Source: CAD feature listing. Evaluate the final solid. Frame: model axes, mm. Face numbers are marked on the shaded views. Round coordinates to 2 decimals unless told otherwise and drop trailing zeros. Loops run counter-clockwise (first coordinate to the right, second up) from the corner with the lowest first, then second, coordinate; pieces in that order, holes last.
Item 1: First-contact query: P1, Ø3, axis at y = -28.5, z = -3, coming from the +X side; P2, Ø8, axis at x = -10.5, y = -26, coming from the +Z side; P3, Ø3, axis at x = 9, y = -29, coming from the +Z side. Flat tips, straight axial feed; report the tip coordinate or a pass-through.
Item 2: Section query A-A on z = 0. Return loops of the section in (x, y).
Item 3: Section query B-B on x = 0. Return loops of the section in (y, z).
Item 4: Section query C-C on y = -27.5. Return loops of the section in (x, z).
Item 5: Pull-direction query (Z, two-part tool) for the marked faces 1, 2 and 3; classes: released by +Z, released by -Z, zero draft, split by the parting line, or undercut.
Item 6: Ray query, L1, parallel to X at y = -27.75, z = 0; L2, parallel to X at y = -24.5, z = 16. Return the intervals inside material, ascending.
```python
from build123d import *

# Parameters (mm, degrees)
RACCORDO1_R  = 4
SMUSSO1_SIZE = 0.5
SMUSSO2_SIZE = 0.3
RACCORDO5_R  = 0.8


with BuildPart() as part:
    # Schizzo1 → Rivoluzione1 (revolve)
    with BuildSketch(Plane.XY):
        Polygon((-34, -19.165655205), (-34, -34.165655205), (-23.25, -34.165655205), (-22.25, -33.465655205), (-20, -33.465655205), (-20, -20.665655205), (-17.75, -20.665655205), (-17.75, -19.165655205), align=None)
    revolve(axis=Axis((0, 44.110898502, 0), (0, -1, 0)))

    # Raccordo1
    raccordo1_edges = [part.edges().sort_by_distance(p)[0] for p in [
        (34, -34.165655205, 0),
        (34, -19.165655205, 0),
    ]]
    fillet(raccordo1_edges, radius=RACCORDO1_R)

    # Smusso1
    smusso1_edges = [part.edges().sort_by_distance(p)[0] for p in [
        (17.75, -19.165655205, 0),
    ]]
    chamfer(smusso1_edges, length=SMUSSO1_SIZE)

    # Smusso2
    smusso2_edges = [part.edges().sort_by_distance(p)[0] for p in [
        (20, -33.465655205, 0),
    ]]
    chamfer(smusso2_edges, length=SMUSSO2_SIZE)

    # Raccordo5
    raccordo5_edges = [part.edges().sort_by_distance(p)[0] for p in [
        (20, -20.665655205, 0),
    ]]
    fillet(raccordo5_edges, radius=RACCORDO5_R)


solid = part.part
```
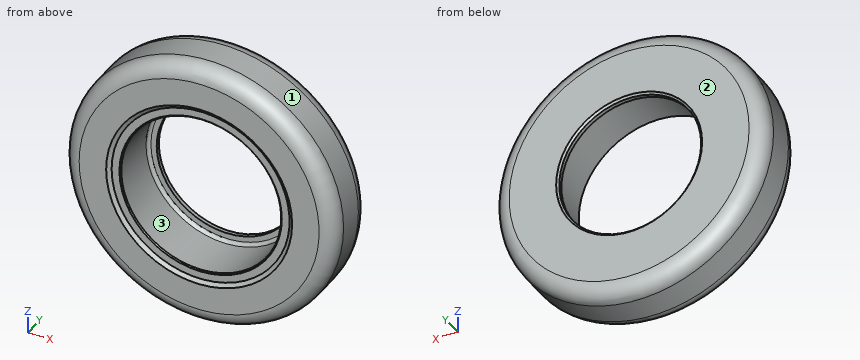
Data:
1. P1: stops at x = 33.97
1. P2: stops at z = 33.37
1. P3: stops at z = 33.16
2. outline: (-34, -30.17) arc R4 ccw to (-30, -34.17) - (-23.25, -34.17) - (-22.25, -33.47) - (-20.3, -33.47) - (-20, -33.17) - (-20, -21.47) arc R0.8 cw to (-19.2, -20.67) - (-17.75, -20.67) - (-17.75, -19.67) - (-18.25, -19.17) - (-30, -19.17) arc R4 ccw to (-34, -23.17) - close; (17.75, -20.67) - (19.2, -20.67) arc R0.8 cw to (20, -21.47) - (20, -33.17) - (20.3, -33.47) - (22.25, -33.47) - (23.25, -34.17) - (30, -34.17) arc R4 ccw to (34, -30.17) - (34, -23.17) arc R4 ccw to (30, -19.17) - (18.25, -19.17) - (17.75, -19.67) - close
3. outline: (-34.17, -30) arc R4 ccw to (-30.17, -34) - (-23.17, -34) arc R4 ccw to (-19.17, -30) - (-19.17, -18.25) - (-19.67, -17.75) - (-20.67, -17.75) - (-20.67, -19.2) arc R0.8 cw to (-21.47, -20) - (-33.17, -20) - (-33.47, -20.3) - (-33.47, -22.25) - (-34.17, -23.25) - close; (-34.17, 23.25) - (-33.47, 22.25) - (-33.47, 20.3) - (-33.17, 20) - (-21.47, 20) arc R0.8 cw to (-20.67, 19.2) - (-20.67, 17.75) - (-19.67, 17.75) - (-19.17, 18.25) - (-19.17, 30) arc R4 ccw to (-23.17, 34) - (-30.17, 34) arc R4 ccw to (-34.17, 30) - close
4. outline: circle Ø68 at (0, 0); hole circle Ø40 at (0, 0)
5. face 1: split by the parting line
5. face 2: zero draft
5. face 3: undercut
6. L1: x = -34 to -20, 20 to 34
6. L2: x = -30 to -12, 12 to 30
